Source: CAD feature listing. Evaluate the final solid. Frame: model axes, mm. Face numbers are marked on the shaded views. A direction names the side the tool comes from. Coordinates: 2 decimals unless noted, no trailing zeros. Loops run counter-clockwise (first coordinate to the right, second up) from the corner with the lowest first, then second, coordinate; pieces in that order, holes last. Notation, with made-up numbers: M 80.25,11 L 84.25,11 A37 ccw 84.25,48 Z; hole C -28.75,-33.5 d1. An arc over 180 degrees is marked long. One line per question, with ' | ' between items. Start each with the question number.
1. Section query C-C, the plane x = 0. Output: boundary loops of the cut face in (y, z), and give its area (3 significant figures).
2. Access query for the marked faces 5, 6 and 7. Directions: +Z, -Z, +X, -X, +Y, -Y. A direction counts if a zero-diameter tool reaches every point of the face in a straight line with its end or side. Return the directions, or none.
3. Section query A-A, the plane y = -18. Output: boundary loops of the cut face in (x, z), and give its area (3 significant figures).
4. Section query B-B, the plane z = -7. Output: boundary loops of the cut face in (x, y), and give its area (3 significant figures).
5. Ray query, probe 1 along Z at (x, y) = (-9, -7.5); probe 2 along X at (y, z) = (-2.5, -3); probe 3 along Y at (x, z) = (-12, -9.45). Return the intervals inside material, ascending.
6. Section query D-D, the plane y = -8.5. Output: boundary loops of the cut face in (x, z).
7. Pin query (flat end, axial travel): P1, Ø4.5, axis at y = 2.5, z = -4.5, coming from the +X side; P2, Ø1, axis at y = 6.5, z = -6, coming from the -X side; P3, Ø1.5, axis at x = -1, y = 9.5, coming from the +Z side. Return the tip coordinate at first contact, or that it passes through.
8. Mould query, pull axis Y, two halves, no side actions, for the marked faces 1, 2, 3 and 4. Classes: pulls with the +Y half, pulls with the -Y half, needs draft (parallel to the pull), parting line crosses it, or undercut.
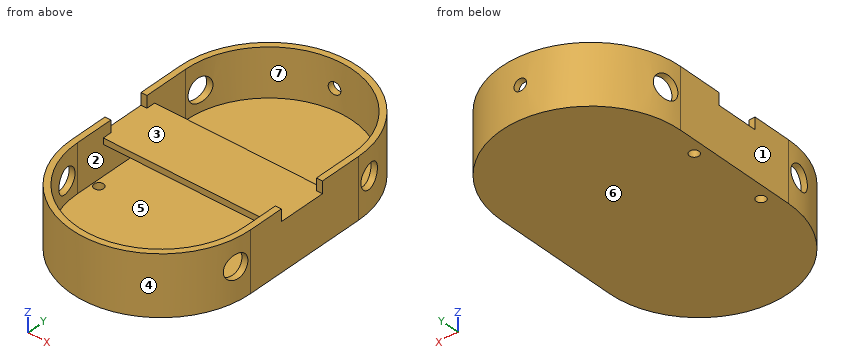
```python
from build123d import *

# Parameters (mm, degrees)
CYLINDER053_R           = 0.8
CYLINDER053_DEPTH       = 10
CYLINDER052_R           = 0.8
CYLINDER052_DEPTH       = 10
BOX056_W                = 1
BOX056_H                = 1
BOX056_DEPTH            = 2
BOX057_W                = 1
BOX057_H                = 1
BOX057_DEPTH            = 2
CYLINDER037_R           = 1
CYLINDER037_DEPTH       = 10
CYLINDER037_ROLL_ANGLE  = 90
CYLINDER029_R           = 2
CYLINDER029_DEPTH       = 10
CYLINDER029_PITCH_ANGLE = 90
CYLINDER031_R           = 2
CYLINDER031_DEPTH       = 10
CYLINDER031_PITCH_ANGLE = 90
CYLINDER030_R           = 2
CYLINDER030_DEPTH       = 10
CYLINDER030_PITCH_ANGLE = 90
CYLINDER028_R           = 2
CYLINDER028_DEPTH       = 10
CYLINDER028_PITCH_ANGLE = 90
BOX012_W                = 33
BOX012_H                = 8
BOX012_DEPTH            = 2
CYLINDER002_W           = 14
CYLINDER002_H           = 8
CYLINDER002_ANGLE       = 180
CYLINDER001_W           = 15
CYLINDER001_H           = 10
CYLINDER001_ANGLE       = 180
CYLINDER003_W           = 14
CYLINDER003_H           = 8
CYLINDER003_ANGLE       = 180
CYLINDER_W              = 15
CYLINDER_H              = 10
CYLINDER_ANGLE          = 180
BOX001_W                = 28
BOX001_H                = 21
BOX001_DEPTH            = 8
BOX_W                   = 30
BOX_H                   = 21
BOX_DEPTH               = 10
FUSION_PLACEMENT_ANGLE  = 180
BOX013_W                = 28
BOX013_H                = 10
BOX013_DEPTH            = 2
BOX011_W                = 28
BOX011_H                = 10
BOX011_DEPTH            = 3


with BuildPart() as cilindro053:
    # Cylinder053 → Cylinder053 (new body)
    with BuildSketch(Plane(origin=(-12, -18, -17), x_dir=(1, 0, 0), z_dir=(0, 0, 1))):
        Circle(CYLINDER053_R)
    extrude(amount=CYLINDER053_DEPTH)


with BuildPart() as cilindro052:
    # Cylinder052 → Cylinder052 (new body)
    with BuildSketch(Plane(origin=(-12, -5, -17), x_dir=(1, 0, 0), z_dir=(0, 0, 1))):
        Circle(CYLINDER052_R)
    extrude(amount=CYLINDER052_DEPTH)


with BuildPart() as cubo056:
    # Box056 → Box056 (new body)
    with BuildSketch(Plane(origin=(-14, -7.5, -2), x_dir=(1, 0, 0), z_dir=(0, 0, 1))):
        with Locations((0.5, 0.5)):
            Rectangle(BOX056_W, BOX056_H)
    extrude(amount=BOX056_DEPTH)


with BuildPart() as cubo057:
    # Box057 → Box057 (new body)
    with BuildSketch(Plane(origin=(-14, -15.5, -2), x_dir=(1, 0, 0), z_dir=(0, 0, 1))):
        with Locations((0.5, 0.5)):
            Rectangle(BOX057_W, BOX057_H)
    extrude(amount=BOX057_DEPTH)


with BuildPart() as cilindro037:
    # Cylinder037 → Cylinder037 (new body)
    with BuildSketch(Plane.XY):
        Circle(CYLINDER037_R)
    extrude(amount=CYLINDER037_DEPTH)


with BuildPart() as cilindro037_1:
    # Cylinder037 roll: moved
    add(cilindro037.part.rotate(Axis((0, 0, 0), (1, 0, 0)), CYLINDER037_ROLL_ANGLE))


with BuildPart() as cilindro037_2:
    # Cylinder037 placement: moved
    add(cilindro037_1.part.moved(Location((-14, 89, 39.5))))


with BuildPart() as cilindro029:
    # Cylinder029 → Cylinder029 (new body)
    with BuildSketch(Plane.XY):
        Circle(CYLINDER029_R)
    extrude(amount=CYLINDER029_DEPTH)


with BuildPart() as cilindro029_1:
    # Cylinder029 pitch: moved
    add(cilindro029.part.rotate(Axis((0, 0, 0), (0, 1, 0)), CYLINDER029_PITCH_ANGLE))


with BuildPart() as cilindro029_2:
    # Cylinder029 placement: moved
    add(cilindro029_1.part.moved(Location((-29, 46.5, 39.5))))


with BuildPart() as cilindro031:
    # Cylinder031 → Cylinder031 (new body)
    with BuildSketch(Plane.XY):
        Circle(CYLINDER031_R)
    extrude(amount=CYLINDER031_DEPTH)


with BuildPart() as cilindro031_1:
    # Cylinder031 pitch: moved
    add(cilindro031.part.rotate(Axis((0, 0, 0), (0, 1, 0)), CYLINDER031_PITCH_ANGLE))


with BuildPart() as cilindro031_2:
    # Cylinder031 placement: moved
    add(cilindro031_1.part.moved(Location((-5, 72.5, 39.5))))


with BuildPart() as cilindro030:
    # Cylinder030 → Cylinder030 (new body)
    with BuildSketch(Plane.XY):
        Circle(CYLINDER030_R)
    extrude(amount=CYLINDER030_DEPTH)


with BuildPart() as cilindro030_1:
    # Cylinder030 pitch: moved
    add(cilindro030.part.rotate(Axis((0, 0, 0), (0, 1, 0)), CYLINDER030_PITCH_ANGLE))


with BuildPart() as cilindro030_2:
    # Cylinder030 placement: moved
    add(cilindro030_1.part.moved(Location((-5, 46.5, 39.5))))


with BuildPart() as cilindro028:
    # Cylinder028 → Cylinder028 (new body)
    with BuildSketch(Plane.XY):
        Circle(CYLINDER028_R)
    extrude(amount=CYLINDER028_DEPTH)


with BuildPart() as cilindro028_1:
    # Cylinder028 pitch: moved
    add(cilindro028.part.rotate(Axis((0, 0, 0), (0, 1, 0)), CYLINDER028_PITCH_ANGLE))


with BuildPart() as cilindro028_2:
    # Cylinder028 placement: moved
    add(cilindro028_1.part.moved(Location((-29, 72.5, 39.5))))


with BuildPart() as cubo012:
    # Box012 → Box012 (new body)
    with BuildSketch(Plane(origin=(-30, 55, 42), x_dir=(1, 0, 0), z_dir=(0, 0, 1))):
        with Locations((16.5, 4)):
            Rectangle(BOX012_W, BOX012_H)
    extrude(amount=BOX012_DEPTH)


with BuildPart() as cilindro002:
    # Cylinder002 → Cylinder002 (revolve)
    with BuildSketch(Plane(origin=(16, 49, -36), x_dir=(1, 0, 0), z_dir=(0, 1, 0))):
        with Locations((7, 4)):
            Rectangle(CYLINDER002_W, CYLINDER002_H)
    revolve(axis=Axis((16, 49, -36), (0, 0, -1)), revolution_arc=CYLINDER002_ANGLE)


with BuildPart() as cut001:
    # Cylinder001 → Cylinder001 (revolve)
    with BuildSketch(Plane(origin=(16, 49, -34), x_dir=(1, 0, 0), z_dir=(0, 1, 0))):
        with Locations((7.5, 5)):
            Rectangle(CYLINDER001_W, CYLINDER001_H)
    revolve(axis=Axis((16, 49, -34), (0, 0, -1)), revolution_arc=CYLINDER001_ANGLE)

    # Cut001: cut Cilindro002
    add(cilindro002.part, mode=Mode.SUBTRACT)


with BuildPart() as cut001_1:
    # Cut001 placement: moved
    add(cut001.part.moved(Location((-3, 0, 0))))


with BuildPart() as cilindro003:
    # Cylinder003 → Cylinder003 (revolve)
    with BuildSketch(Plane(origin=(13, 70, -36), x_dir=(-1, 0, 0), z_dir=(0, -1, 0))):
        with Locations((7, 4)):
            Rectangle(CYLINDER003_W, CYLINDER003_H)
    revolve(axis=Axis((13, 70, -36), (0, 0, -1)), revolution_arc=CYLINDER003_ANGLE)


with BuildPart() as cut002:
    # Cylinder → Cylinder (revolve)
    with BuildSketch(Plane(origin=(13, 70, -34), x_dir=(-1, 0, 0), z_dir=(0, -1, 0))):
        with Locations((7.5, 5)):
            Rectangle(CYLINDER_W, CYLINDER_H)
    revolve(axis=Axis((13, 70, -34), (0, 0, -1)), revolution_arc=CYLINDER_ANGLE)

    # Cut002: cut Cilindro003
    add(cilindro003.part, mode=Mode.SUBTRACT)


with BuildPart() as cubo001:
    # Box001 → Box001 (new body)
    with BuildSketch(Plane(origin=(-1, 49, -44), x_dir=(1, 0, 0), z_dir=(0, 0, 1))):
        with Locations((14, 10.5)):
            Rectangle(BOX001_W, BOX001_H)
    extrude(amount=BOX001_DEPTH)


with BuildPart() as cut058:
    # Box → Box (new body)
    with BuildSketch(Plane(origin=(-2, 49, -44), x_dir=(1, 0, 0), z_dir=(0, 0, 1))):
        with Locations((15, 10.5)):
            Rectangle(BOX_W, BOX_H)
    extrude(amount=BOX_DEPTH)

    # Cut: cut Cubo001
    add(cubo001.part, mode=Mode.SUBTRACT)

    # Fusion: union Cut001, Cut002
    add(cut001_1.part)
    add(cut002.part)


with BuildPart() as cut058_1:
    # Fusion placement: moved
    add(cut058.part.rotate(Axis((0, 0, 0), (0, 1, 0)), FUSION_PLACEMENT_ANGLE))

    # Cut003: cut Cubo012
    add(cubo012.part, mode=Mode.SUBTRACT)

    # Cut040: cut Cilindro028
    add(cilindro028_2.part, mode=Mode.SUBTRACT)

    # Cut041: cut Cilindro030
    add(cilindro030_2.part, mode=Mode.SUBTRACT)

    # Cut042: cut Cilindro031
    add(cilindro031_2.part, mode=Mode.SUBTRACT)

    # Cut043: cut Cilindro029
    add(cilindro029_2.part, mode=Mode.SUBTRACT)

    # Cut058: cut Cilindro037
    add(cilindro037_2.part, mode=Mode.SUBTRACT)


with BuildPart() as cubo013:
    # Box013 → Box013 (new body)
    with BuildSketch(Plane(origin=(-27, 54, 42), x_dir=(1, 0, 0), z_dir=(0, 0, 1))):
        with Locations((14, 5)):
            Rectangle(BOX013_W, BOX013_H)
    extrude(amount=BOX013_DEPTH)


with BuildPart() as cut077:
    # Box011 → Box011 (new body)
    with BuildSketch(Plane(origin=(-27, 54, 41), x_dir=(1, 0, 0), z_dir=(0, 0, 1))):
        with Locations((14, 5)):
            Rectangle(BOX011_W, BOX011_H)
    extrude(amount=BOX011_DEPTH)

    # Cut004: cut Cubo013
    add(cubo013.part, mode=Mode.SUBTRACT)

    # Fusion002022: union Cut058
    add(cut058_1.part)


with BuildPart() as cut077_1:
    # Fusion002022 placement: moved
    add(cut077.part.moved(Location((14, -70, -44))))

    # Fusion002031: union Cubo056, Cubo057
    add(cubo056.part)
    add(cubo057.part)

    # Cut076: cut Cilindro052
    add(cilindro052.part, mode=Mode.SUBTRACT)

    # Cut077: cut Cilindro053
    add(cilindro053.part, mode=Mode.SUBTRACT)


solid = cut077_1.part
```
Taken from the geometry:
1) outline: M -35.97,-10 L 14.97,-10 L 14.97,-5.5 L 13.96,-5.5 L 13.96,-8 L -34.96,-8 L -34.96,0 L -35.97,0 Z; M -16,-3 L -6,-3 L -6,-2 L -16,-2 Z; M 13.96,-3.5 L 14.97,-3.5 L 14.97,0 L 13.96,0 Z | area: 126 mm^2
2) face 5: none | face 6: -Z, +X, -X, +Y, -Y | face 7: +Z
3) outline: M -14,-10 L -12.8,-10 L -12.8,-8 L -13,-8 L -13,0 L -14,0 Z; M -11.2,-10 L 16,-10 L 16,0 L 15,0 L 15,-8 L -11.2,-8 Z | area: 72.8 mm^2
4) outline: M -14,-21 A15 ccw 16,-21 L 16,0 A15 ccw -14,0 Z; hole M -13,-21 A14 ccw 15,-21 L 15,0 A14 ccw -13,0 Z | area: 133 mm^2
5) probe 1: -10 to -8, -3 to -2 | probe 2: -14 to -13, 15 to 16 | probe 3: -28.48 to -18.8, -17.2 to -5.8, -4.2 to 7.48
6) outline: M -14,-10 L 16,-10 L 16,-2 L -14,-2 Z; hole M -13,-8 L 15,-8 L 15,-3 L -13,-3 Z
7) P1: x = 16 | P2: x = -12.75 | P3: z = -8
8) face 1: needs draft | face 2: undercut | face 3: undercut | face 4: pulls with the -Y half
